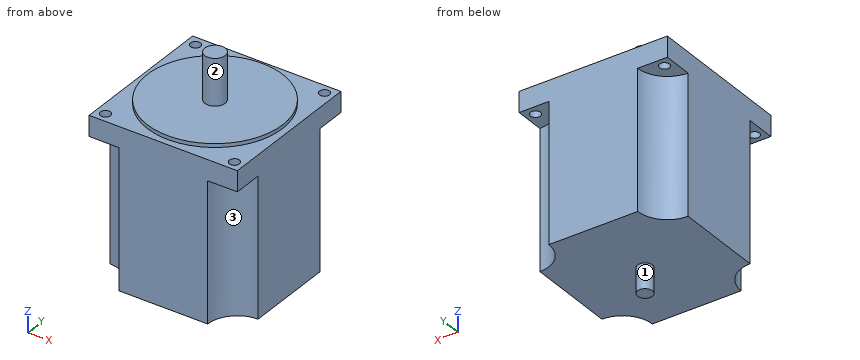
```python
from build123d import *

# Parameters (mm, degrees)
SKETCH2_W           = 80
SKETCH2_H           = 80
BOSS_EXTRUDE1_DEPTH = 86.09
SKETCH3_R           = 2.75
CUT_EXTRUDE1_DEPTH  = 104.012077447
SKETCH4_R           = 36.5
BOSS_EXTRUDE2_DEPTH = 2
SKETCH5_R           = 5.5
BOSS_EXTRUDE3_DEPTH = 25
CUT_EXTRUDE2_START  = -75
SKETCH6_R           = 2.75
CUT_EXTRUDE2_DEPTH  = 75
SKETCH7_R           = 4.006
BOSS_EXTRUDE4_DEPTH = 13.5


with BuildPart() as part:
    # Sketch2 → Boss-Extrude1 (new body)
    with BuildSketch(Plane.XY):
        Rectangle(SKETCH2_W, SKETCH2_H)
    extrude(amount=BOSS_EXTRUDE1_DEPTH)

    # Sketch3 → Cut-Extrude1 (cut, through all)
    with BuildSketch(Plane.XY.offset(86.09)):
        with Locations((-34.8, 34.8)):
            Circle(SKETCH3_R)
        with Locations((34.8, 34.8)):
            Circle(SKETCH3_R)
        with Locations((-34.8, -34.8)):
            Circle(SKETCH3_R)
        with Locations((34.8, -34.8)):
            Circle(SKETCH3_R)
    extrude(amount=-CUT_EXTRUDE1_DEPTH, mode=Mode.SUBTRACT)

    # Sketch4 → Boss-Extrude2 (add)
    with BuildSketch(Plane.XY.offset(86.09)):
        Circle(SKETCH4_R)
    extrude(amount=BOSS_EXTRUDE2_DEPTH)

    # Sketch5 → Boss-Extrude3 (add)
    with BuildSketch(Plane.XY.offset(88.09)):
        Circle(SKETCH5_R)
    extrude(amount=BOSS_EXTRUDE3_DEPTH)

    # Sketch6 → Cut-Extrude2 (cut)
    # profile 1 of 4: a face of its own
    with BuildSketch(Plane(origin=(0, 0, 0), x_dir=(-1, 0, 0), z_dir=(0, 0, -1)).offset(CUT_EXTRUDE2_START)):
        with BuildLine():
            Line((-40, 40), (-40, 24))
            ThreePointArc((-40, 24), (-28.686291501, 28.686291501), (-24, 40))
            Line((-24, 40), (-40, 40))
        make_face()
        with Locations(Location((-34.8, 34.8, 0), (0, 0, 180))):
            Circle(SKETCH6_R, mode=Mode.SUBTRACT)
    # profile 2 of 4: a face of its own
    with BuildSketch(Plane(origin=(0, 0, 0), x_dir=(-1, 0, 0), z_dir=(0, 0, -1)).offset(CUT_EXTRUDE2_START)):
        with BuildLine():
            ThreePointArc((24, 40), (28.686291501, 28.686291501), (40, 24))
            Line((40, 24), (40, 40))
            Line((40, 40), (24, 40))
        make_face()
        with Locations(Location((34.8, 34.8, 0), (0, 0, 180))):
            Circle(SKETCH6_R, mode=Mode.SUBTRACT)
    # profile 3 of 4: a face of its own
    with BuildSketch(Plane(origin=(0, 0, 0), x_dir=(-1, 0, 0), z_dir=(0, 0, -1)).offset(CUT_EXTRUDE2_START)):
        with BuildLine():
            Line((24, -40), (40, -40))
            Line((40, -40), (40, -24))
            ThreePointArc((40, -24), (28.686291501, -28.686291501), (24, -40))
        make_face()
        with Locations(Location((34.8, -34.8, 0), (0, 0, 180))):
            Circle(SKETCH6_R, mode=Mode.SUBTRACT)
    # profile 4 of 4: a face of its own
    with BuildSketch(Plane(origin=(0, 0, 0), x_dir=(-1, 0, 0), z_dir=(0, 0, -1)).offset(CUT_EXTRUDE2_START)):
        with BuildLine():
            Line((-40, -40), (-24, -40))
            ThreePointArc((-24, -40), (-28.686291501, -28.686291501), (-40, -24))
            Line((-40, -24), (-40, -40))
        make_face()
        with Locations(Location((-34.8, -34.8, 0), (0, 0, 180))):
            Circle(SKETCH6_R, mode=Mode.SUBTRACT)
    extrude(amount=CUT_EXTRUDE2_DEPTH, mode=Mode.SUBTRACT)

    # Sketch7 → Boss-Extrude4 (add)
    with BuildSketch(Plane(origin=(0, 0, 0), x_dir=(-1, 0, 0), z_dir=(0, 0, -1))):
        with Locations(Location((0, 0, 0), (0, 0, 180))):
            Circle(SKETCH7_R)
    extrude(amount=BOSS_EXTRUDE4_DEPTH)


solid = part.part
```
Work out the finished part from the listing and answer in its coordinate system (mm). Face numbers are marked on the shaded views. A direction names the side the tool comes from. Give positions to 0.01 mm unless a question says otherwise; leave off trailing zeros. Loops run counter-clockwise (first coordinate to the right, second up) from the corner with the lowest first, then second, coordinate; pieces in that order, holes last. Notation, with made-up numbers: M 29.5,86.25 L 71.5,86.25 A26 cw 71.5,109.25 Z; hole C 36.25,4.25 d3. An arc over 180 degrees is marked long. One line per item, written item: value. Start each with the question number.
1. Find section A-A (z = 12). Give the vertices of the cut face in (x, y).
2. Find section B-B (x = -34.8). Give the vertices of the cut face in (y, z).
3. Find section C-C (x = 0). Give the vertices of the cut face in (y, z), and give its area (3 significant figures).
4. Which of the six approach directions +Z, -Z, +X, -X, +Y, -Y give full straight-line access (tool end or side, diameter ignored) to the marked faces 1, 2 and 3?
5. Find the intervals of material crossed by probe 1 along X at (y, z) = (34.8, 78); probe 2 along X at (y, z) = (-34, 83), in increasing order.
6. Each of these flat-tipped pins is pushed along its axis until it touches: P1, Ø5, axis at x = 12.5, y = -16, coming from the +Z side; P2, Ø13, axis at x = 31.5, y = 32, coming from the -Z side; P3, Ø7, axis at x = 34.8, y = -34.8, coming from the +Z side. Where does it stop, or does it pass through?
Reported:
1. outline: M -40,-24 A16 cw -24,-40 L 24,-40 A16 cw 40,-24 L 40,24 A16 cw 24,40 L -24,40 A16 cw -40,24 Z
2. outline: M -40,75 L -37.55,75 L -37.55,86.09 L -40,86.09 Z; M -32.05,75 L -24.87,75 L -24.87,0 L 24.87,0 L 24.87,75 L 32.05,75 L 32.05,86.09 L 11.01,86.09 L 11.01,88.09 L -11.01,88.09 L -11.01,86.09 L -32.05,86.09 Z; M 37.55,75 L 40,75 L 40,86.09 L 37.55,86.09 Z
3. outline: M -40,0 L -4.01,0 L -4.01,-13.5 L 4.01,-13.5 L 4.01,0 L 40,0 L 40,86.09 L 36.5,86.09 L 36.5,88.09 L 5.5,88.09 L 5.5,113.09 L -5.5,113.09 L -5.5,88.09 L -36.5,88.09 L -36.5,86.09 L -40,86.09 Z
3. area: 7,420 mm²
4. face 1: -Z
4. face 2: +Z
4. face 3: -Z, +X, -Y
5. probe 1: x = -40 to -37.55, -32.05 to 32.05, 37.55 to 40
5. probe 2: x = -40 to -37.43, -32.17 to 32.17, 37.43 to 40
6. P1: stops at z = 88.09
6. P2: stops at z = 0
6. P3: stops at z = 86.09
